Part model, mm, in its own coordinate system. A direction names the side the tool comes from. Round coordinates to 2 decimals unless told otherwise and drop trailing zeros. Loops run counter-clockwise (first coordinate to the right, second up) from the corner with the lowest first, then second, coordinate; pieces in that order, holes last. Notation, with made-up numbers: (7.5, 83) - (44.5, 83) arc R28 cw to (44.5, 104) - close; hole circle Ø8 at (12, -29.75). An arc over 180 degrees is marked (long way). Put each result on its own line as item: value.
from build123d import *

# Parameters (mm, degrees)
F0_W     = 238.8686686754
F0_H     = 158.1714600325
F1_DEPTH = 68.326
F2_T     = -2.54
F3_R     = 5.08


with BuildPart() as f1:
    # F0 (on Front) → F1 (new body)
    with BuildSketch(Plane.XZ):
        Rectangle(F0_W, F0_H)
    extrude(amount=F1_DEPTH)

    # F2
    f2_openings = [f1.faces().sort_by_distance(p)[0] for p in [
        (0, -68.326, 0),
    ]]
    offset(amount=F2_T, openings=f2_openings)

    # F3
    f3_edges = [f1.edges().sort_by_distance(p)[0] for p in [
        (-119.434334, -34.163, 79.08573),
        (119.434334, -34.163, 79.08573),
        (119.434334, -34.163, -79.08573),
        (-116.894334, -35.433, -76.54573),
    ]]
    fillet(f3_edges, radius=F3_R)


solid = f1.part
1. Two-plate mould, pull along Z, no slides. Class faces 1 (the flat face through (-119.434, -34, -4)), 2 (the flat face through (-2, -34, 79.086)), 3 (the flat face through (1, -35, -76.546)): pulls with the +Z half, pulls with the -Z half, needs draft (parallel to the pull), parting line crosses it, or undercut.
A:
face 1: needs draft
face 2: pulls with the +Z half
face 3: undercut
2. Pin check, flat tips, straight feed: P1, Ø6, axis at x = 66.5, z = -14, coming from the -Y side; P2, Ø4, axis at x = -77, z = -41, coming from the +Y side. Stop position of each tip, or through.
A:
P1: stops at y = -2.54
P2: stops at y = 0
3. Band-saw the part on B-B (z = -46.5). List the corners of the cut face in (x, y), plus the area to 3 significant figures.
A:
outline: (-119.43, -68.33) - (-116.89, -68.33) - (-116.89, -2.54) - (116.89, -2.54) - (116.89, -68.33) - (119.43, -68.33) - (119.43, 0) - (-119.43, 0) - close
area: 941 mm²
4. Band-saw the part on A-A (y = -44.5). List the corners of the cut face in (x, z).
A:
outline: (-119.43, -79.09) - (114.35, -79.09) arc R5.08 ccw to (119.43, -74.01) - (119.43, 74.01) arc R5.08 ccw to (114.35, 79.09) - (-114.35, 79.09) arc R5.08 ccw to (-119.43, 74.01) - close; hole (-116.89, -71.47) arc R5.08 ccw to (-111.81, -76.55) - (116.89, -76.55) - (116.89, 76.55) - (-116.89, 76.55) - close
5. Probe line 1 along Z through (x, y) = (-22.5, -41); line 2 along X through (y, z) = (-52, 9.5); line 3 along Y through (x, z) = (103, -48.5). List the from-to ranges inside material, lowest first. Write a range as [from, to].
A:
line 1: z = [-79.09, -76.55], [76.55, 79.09]
line 2: x = [-119.43, -116.89], [116.89, 119.43]
line 3: y = [-2.54, 0]
6. Band-saw the part on C-C (x = 18.5). List the corners of the cut face in (y, z).
A:
outline: (-68.33, -79.09) - (0, -79.09) - (0, 79.09) - (-68.33, 79.09) - (-68.33, 76.55) - (-2.54, 76.55) - (-2.54, -76.55) - (-68.33, -76.55) - close
7. Tool access for faces 4 (the flat face through (-2, -35, 76.546)), 5 (the cylindrical face through (-117.986, -34.641, 77.558)): list every direction of +Z, -Z, +X, -X, +Y, -Y with a clear straight run to the whole face (end or side of a thin tool).
A:
face 4: -Y
face 5: +Z, -X, +Y, -Y
